For this review, take the finished solid that the model builds, in its own axes (mm). A direction names the side the tool comes from. Coordinates: 2 decimals unless noted, no trailing zeros. Write each loop counter-clockwise with the first axis right and the second up, starting at its lowest first coordinate (ties: lowest second). Pieces come first, ordered by that corner, then holes.
```python
from build123d import *

# Parameters (mm, degrees)
BOSS_EXTRUDE1_DEPTH = 139.7
SKETCH2_W           = 25.4
SKETCH2_H           = 31.75
BOSS_EXTRUDE2_DEPTH = 3.175
SKETCH3_W           = 3.175
SKETCH3_H           = 31.75
BOSS_EXTRUDE3_DEPTH = 25.4
SKETCH5_W           = 22.225
SKETCH5_H           = 3.175
SKETCH5_W_2         = 25.4
SKETCH5_H_2         = 25.4
SKETCH5_H_3         = 22.225
BOSS_EXTRUDE4_DEPTH = 31.75


with BuildPart() as part:
    # Sketch1 → Boss-Extrude1 (new body)
    with BuildSketch(Plane(origin=(0, 0, 0), x_dir=(0, 0, -1), z_dir=(1, 0, 0))):
        Polygon((-31.75, 0), (0, 0), (0, 31.75), (6.35, 31.75), (6.35, -6.35), (-31.75, -6.35), align=None)
    extrude(amount=BOSS_EXTRUDE1_DEPTH)

    # Sketch2 → Boss-Extrude2 (add)
    with BuildSketch(Plane(origin=(0, 0, 0), x_dir=(1, 0, 0), z_dir=(0, 1, 0))):
        with Locations((12.7, -15.875)):
            Rectangle(SKETCH2_W, SKETCH2_H)
        with Locations((127, -15.875)):
            Rectangle(SKETCH2_W, SKETCH2_H)
    extrude(amount=BOSS_EXTRUDE2_DEPTH)

    # Sketch3 → Boss-Extrude3 (add)
    with BuildSketch(Plane(origin=(0, 3.175, 0), x_dir=(1, 0, 0), z_dir=(0, 1, 0))):
        with Locations((23.8125, -15.875)):
            Rectangle(SKETCH3_W, SKETCH3_H)
        with Locations((115.8875, -15.875)):
            Rectangle(SKETCH3_W, SKETCH3_H)
    extrude(amount=BOSS_EXTRUDE3_DEPTH)

    # Sketch5 → Boss-Extrude4 (add)
    # profile 1 of 8: a face of its own
    with BuildSketch(Plane.XY):
        Polygon((19.05, 7.657352941), (22.225, 7.657352941), (22.225, 29.882352941), (22.225, 33.057352941), (19.05, 33.057352941), align=None)
    # profile 2 of 8: a face of its own
    with BuildSketch(Plane.XY):
        with Locations((33.3375, 31.469852941)):
            Rectangle(SKETCH5_W, SKETCH5_H)
    # profile 3 of 8: a face of its own
    with BuildSketch(Plane.XY):
        Polygon((19.05, 34.644852941), (19.05, 33.057352941), (22.225, 33.057352941), (44.45, 33.057352941), (95.25, 33.057352941), (117.475, 33.057352941), (120.65, 33.057352941), (120.65, 34.644852941), (84.1375, 34.644852941), (82.55, 34.644852941), (57.15, 34.644852941), (55.5625, 34.644852941), align=None)
    # profile 4 of 8: a face of its own
    with BuildSketch(Plane.XY):
        Polygon((55.5625, 63.026302863), (55.5625, 34.644852941), (57.15, 34.644852941), (57.15, 60.044852941), (57.15, 63.219852941), (47.625, 101.701283211), (46.084004478, 101.319852941), align=None)
    # profile 5 of 8: a face of its own
    with BuildSketch(Plane.XY):
        with Locations((106.3625, 31.469852941)):
            Rectangle(SKETCH5_W, SKETCH5_H)
    # profile 6 of 8: a face of its own
    with BuildSketch(Plane.XY):
        with Locations((69.85, 47.344852941)):
            Rectangle(SKETCH5_W_2, SKETCH5_H_2)
        with Locations((69.85, 47.344852941)):
            Rectangle(SKETCH5_W, SKETCH5_H_3, mode=Mode.SUBTRACT)
    # profile 7 of 8: a face of its own
    with BuildSketch(Plane.XY):
        Polygon((120.65, 33.057352941), (117.475, 33.057352941), (117.475, 29.882352941), (117.475, 7.657352941), (120.65, 7.657352941), align=None)
    # profile 8 of 8: a face of its own
    with BuildSketch(Plane.XY):
        Polygon((82.55, 60.044852941), (82.55, 34.644852941), (84.1375, 34.644852941), (84.1375, 63.026302863), (93.615995522, 101.319852941), (92.075, 101.701283211), (82.55, 63.219852941), align=None)
    extrude(amount=BOSS_EXTRUDE4_DEPTH)


solid = part.part
```
Q1. Draft analysis for pull direction X (two halves, no side actions). For faces 1 (the flat face through (58, 49, 0)), 2 (the flat face through (69, 33.057, 16)), 3 (the flat face through (55.562, 49, 16)), state which applies: +X half, -X half, draft (parallel to the pull), parting line (faces both ways), or undercut.
Ans:
face 1: draft
face 2: undercut
face 3: -X half
Q2. Add section B-B (x = 100). State the section outline as (y, z) points, then the cut area to 3 significant figures.
Ans:
outline: (-6.35, -6.35) - (31.75, -6.35) - (31.75, 0) - (34.64, 0) - (34.64, 31.75) - (29.88, 31.75) - (29.88, 0) - (0, 0) - (0, 31.75) - (-6.35, 31.75) - close
area: 595 mm2
Q3. Add section D-D (y = 21). State the section outline as (x, z) points.
Ans:
outline: (0, -6.35) - (139.7, -6.35) - (139.7, 0) - (120.65, 0) - (120.65, 31.75) - (114.3, 31.75) - (114.3, 0) - (25.4, 0) - (25.4, 31.75) - (19.05, 31.75) - (19.05, 0) - (0, 0) - close
Q4. For probe 1 along Y at (x, z) = (69, 3); probe 2 along Y at (x, z) = (119.5, 9.5) (3 decimals); probe 3 along X at (y, z) = (60.5, 3), list the stretches that pass through material, from the lowest coordinate up.
Ans:
probe 1: y = -6.35 to 0, 33.06 to 36.23, 58.46 to 60.04
probe 2: y = -6.35 to 3.175, 7.657 to 34.645
probe 3: x = 55.56 to 57.15, 82.55 to 84.14
Q5. Add section C-C (x = 53). State the section outline as (y, z) points, then the cut area to 3 significant figures.
Ans:
outline: (-6.35, -6.35) - (31.75, -6.35) - (31.75, 0) - (0, 0) - (0, 31.75) - (-6.35, 31.75) - close; (33.06, 0) - (34.64, 0) - (34.64, 31.75) - (33.06, 31.75) - close; (73.38, 0) - (79.99, 0) - (79.99, 31.75) - (73.38, 31.75) - close
area: 704 mm2
Q6. Clearance check with flat-ended pins moving along their axes: pin 1 Ø11 at (x, z) = (9.5, 18.5) entering from +Y (3 decimals); pin 2 Ø2 at (y, z) = (25, 27) entering from +X; pin 3 Ø14 at (y, z) = (51, 20.5) entering from +X. State where each tip first meets the part, or that it passes through.
Ans:
pin 1: stops at y = 3.175
pin 2: stops at x = 120.65
pin 3: stops at x = 84.14
Q7. Add section A-A (y = 55.5). State the section outline as (x, z) points.
Ans:
outline: (55.56, 0) - (58.74, 0) - (58.74, 31.75) - (55.56, 31.75) - close; (80.96, 0) - (84.14, 0) - (84.14, 31.75) - (80.96, 31.75) - close
Q8. Tool access review of faces 4 (the flat face through (82.55, 62, 16)), 5 (the flat face through (19.05, 21, 16)), 6 (the flat face through (114.3, 14, 16)): name each direction out of +Z, -Z, +X, -X, +Y, -Y from which nothing blocks a thin tool from reaching the whole face with its end or side.
Ans:
face 4: +Z, -Z, +Y
face 5: +Z, -X, +Y
face 6: +Z
